from build123d import *

# Parameters (mm, degrees)
F0_R     = 10.886435
F1_DEPTH = 2
F2_R     = 3.975
F3_DEPTH = 5
F4_R     = 3.15
F5_DEPTH = 4


with BuildPart() as f1:
    # F0 (on Front) → F1 (new body)
    with BuildSketch(Plane.XZ):
        Circle(F0_R)
    extrude(amount=F1_DEPTH)

    # F2 (on face) → F3 (join)
    with BuildSketch(Plane(origin=(0, 0, 0), x_dir=(-1, 0, 0), z_dir=(0, 1, 0))):
        Circle(F2_R)
    extrude(amount=F3_DEPTH)

    # F4 (on face) → F5 (cut)
    with BuildSketch(Plane(origin=(0, 5, 0), x_dir=(-1, 0, 0), z_dir=(0, 1, 0))):
        Circle(F4_R)
    extrude(amount=-F5_DEPTH, mode=Mode.SUBTRACT)


solid = f1.part
The listing builds one solid part. Answer for the finished solid, in the listing's coordinates (mm). A direction names the side the tool comes from. Coordinates: 2 decimals unless noted, no trailing zeros. Loops run counter-clockwise (first coordinate to the right, second up) from the corner with the lowest first, then second, coordinate; pieces in that order, holes last. Notation, with made-up numbers: (10, 41.5) -> (66, 41.5) arc R3 cw to (66, 46.5) -> close; hole circle Ø4 at (34.5, 39.25). An arc over 180 degrees is marked (long way). Answer in a Markdown table with one row per item. Add a question column.
1. Consider line 1 (Z direction, x = 0, y = 2.5) (3 decimals); line 2 (Y direction, x = 9.75, z = 2); line 3 (Z direction, x = 2.25, y = 3). Determine where each line is inside the solid, lowest interval first. Write a range as [from, to].
2. The part is cut by section B-B, the plane z = 0. Write down the section's boundary in (x, y) (3 decimals).
3. Determine the mould class of faces 3 (the flat face through (3, 5, 2)), 4 (the cylindrical face through (10.384, -0.986, 3.27)), 5 (the flat face through (0, 1, 0)) for opening direction Z: +Z half, -Z half, draft (parallel to the pull), parting line (faces both ways), or undercut.
4. For faces 1 (the cylindrical face through (0.86, 2.46, -3.88)), 2 (the flat face through (0, -2, 0)), determine the directions among +Z, -Z, +X, -X, +Y, -Y from which every point of the face is accessible in a straight line to the end or side of a thin tool.
5. The part is cut by section A-A, the plane y = 2.5. Write down the section's boundary in (x, z) (3 decimals), then the cut area to 3 significant figures.
6. The part is cut by section C-C, the plane x = 0. Write down the section's boundary in (y, z) (3 decimals).
7. The part is cut by section D-D, the plane z = 7.25. Write down the section's boundary in (x, y).
8. Flat-ended cylindrical pins translate along their axes: P1, Ø3, axis at x = 0.5, z = 0, coming from the +Y side; P2, Ø1.5, axis at y = -1, z = 3.5, coming from the +X side. Find the tip coordinate at first contact, or state that the pin passes through.
Answer below:
| question | item | result |
|---|---|---|
| 1 | line 1 | [-3.975, -3.15], [3.15, 3.975] |
| 1 | line 2 | [-2, 0] |
| 1 | line 3 | [-3.28, -2.2], [2.2, 3.28] |
| 2 | outline | (-10.886, -2) -> (10.886, -2) -> (10.886, 0) -> (3.975, 0) -> (3.975, 5) -> (3.15, 5) -> (3.15, 1) -> (-3.15, 1) -> (-3.15, 5) -> (-3.975, 5) -> (-3.975, 0) -> (-10.886, 0) -> close |
| 3 | face 3 | draft |
| 3 | face 4 | parting line |
| 3 | face 5 | undercut |
| 4 | face 1 | +Y |
| 4 | face 2 | +Z, -Z, +X, -X, -Y |
| 5 | outline | circle Ø7.95 at (0, 0); hole circle Ø6.3 at (0, 0) |
| 5 | area | 18.5 mm2 |
| 6 | outline | (-2, -10.886) -> (0, -10.886) -> (0, -3.975) -> (5, -3.975) -> (5, -3.15) -> (1, -3.15) -> (1, 3.15) -> (5, 3.15) -> (5, 3.975) -> (0, 3.975) -> (0, 10.886) -> (-2, 10.886) -> close |
| 7 | outline | (-8.12, -2) -> (8.12, -2) -> (8.12, 0) -> (-8.12, 0) -> close |
| 8 | P1 | y = 1 |
| 8 | P2 | x = 10.53 |
